Source: CAD feature listing. Evaluate the final solid. Frame: model axes, mm. Face numbers are marked on the shaded views. A direction names the side the tool comes from. Give positions to 0.01 mm unless a question says otherwise; leave off trailing zeros. Order: outer loops, then holes, each group sorted by start corner. A loop starts at its lowest first (then second) coordinate and runs counter-clockwise, first axis right, second up. Notation, with made-up numbers: M 55.25,18.5 L 85.25,18.5 A7 ccw 85.25,22.5 Z; hole C 1.5,57.5 d4. An arc over 180 degrees is marked long. Answer in a Markdown table with one row per item. Add a question column.
(1) Material intervals for line 1 along Y through (x, z) = (10, 4); line 2 along Y through (x, z) = (5.5, 7.25); line 3 along X through (y, z) = (-3.5, 5.75), sorted ascending.
(2) Mould query, pull axis Y, two halves, no side actions, for the marked faces 1, 2 and 3. Classes: pulls with the +Y half, pulls with the -Y half, needs draft (parallel to the pull), parting line crosses it, or undercut.
(3) Set-up query: the marked faces 4 and 5. Return all of +Z, -Z, +X, -X, +Y, -Y with unobstructed straight access to the full face (end or side cutting, diameter ignored); none if empty.
(4) Section query B-B, the plane x = -3.5. Return loops of the section in (y, z).
(5) Section query D-D, the plane x = -11.25. Return loops of the section in (y, z), plus the area to 3 significant figures.
(6) Section query C-C, the plane y = 12. Return loops of the section in (x, z).
(7) Pin query (flat end, axial travel): P1, Ø2.5, axis at x = 12, y = 12, coming from the -Z side. Return the tip coordinate at first contact, or that it passes through.
(8) Section query A-A, the plane z = 5. Return loops of the section in (x, y).
from build123d import *

# Parameters (mm, degrees)
F0_W     = 30
F0_H     = 30
F0_R     = 1.6
F1_DEPTH = 10.2


with BuildPart() as f1:
    # F0 (on Top) → F1 (new body)
    with BuildSketch(Plane.XY):
        Rectangle(F0_W, F0_H)
        with Locations((-12, -12)):
            Circle(F0_R, mode=Mode.SUBTRACT)
        with Locations((12, -12)):
            Circle(F0_R, mode=Mode.SUBTRACT)
        with Locations((-12, 12)):
            Circle(F0_R, mode=Mode.SUBTRACT)
        with BuildLine():
            ThreePointArc((13.0274698164, 6.366712667), (14.1270717478, 3.2673909823), (14.5, 0))
            ThreePointArc((14.5, 0), (10.6007075236, -9.8931794687), (1, -14.4654761415))
            Line((1, -14.4654761415), (1, -14.5))
            Line((1, -14.5), (0, -14.5))
            Line((0, -14.5), (-1, -14.5))
            Line((-1, -14.5), (-1, -14.4654761415))
            ThreePointArc((-1, -14.4654761415), (-12.5573683549, -7.25), (-13.0274698164, 6.366712667))
            Line((-13.0274698164, 6.366712667), (-13.0573683549, 6.3839745962))
            Line((-13.0573683549, 6.3839745962), (-12.5573697637, 7.2499975598))
            Line((-12.5573697637, 7.2499975598), (-12.0573683549, 8.1160254038))
            Line((-12.0573683549, 8.1160254038), (-12.0274698164, 8.0987634745))
            ThreePointArc((-12.0274698164, 8.0987634745), (0, 14.5), (12.0274698164, 8.0987634745))
            Line((12.0274698164, 8.0987634745), (12.0573683549, 8.1160254038))
            Line((12.0573683549, 8.1160254038), (12.5573697634, 7.2499975604))
            Line((12.5573697634, 7.2499975604), (13.0573683549, 6.3839745962))
            Line((13.0573683549, 6.3839745962), (13.0274698164, 6.366712667))
        make_face(mode=Mode.SUBTRACT)
        with Locations((12, 12)):
            Circle(F0_R, mode=Mode.SUBTRACT)
        with BuildLine():
            Line((6.9371965948, 2.850491783), (13.0274698164, 6.366712667))
            ThreePointArc((13.0274698164, 6.366712667), (12.8000410988, 6.8124113109), (12.5573697634, 7.2499975604))
            ThreePointArc((12.5573697634, 7.2499975604), (12.2997432975, 7.678952716), (12.0274698164, 8.0987634745))
            Line((12.0274698164, 8.0987634745), (5.9371965948, 4.5825425906))
            ThreePointArc((5.9371965948, 4.5825425906), (6.4951905284, 3.75), (6.9371965948, 2.850491783))
        make_face()
        with BuildLine():
            Line((-5.9371965948, 4.5825425906), (-12.0274698164, 8.0987634745))
            ThreePointArc((-12.0274698164, 8.0987634745), (-12.2997432977, 7.6789527158), (-12.5573697637, 7.2499975598))
            ThreePointArc((-12.5573697637, 7.2499975598), (-12.800041099, 6.8124113106), (-13.0274698164, 6.366712667))
            Line((-13.0274698164, 6.366712667), (-6.9371965948, 2.850491783))
            ThreePointArc((-6.9371965948, 2.850491783), (-6.4951905284, 3.75), (-5.9371965948, 4.5825425906))
        make_face()
        with BuildLine():
            ThreePointArc((0, -14.5), (0.5002978855, -14.4913664651), (1, -14.4654761415))
            Line((1, -14.4654761415), (1, -7.4330343737))
            ThreePointArc((1, -7.4330343737), (0, -7.5), (-1, -7.4330343737))
            Line((-1, -7.4330343737), (-1, -14.4654761415))
            ThreePointArc((-1, -14.4654761415), (-0.5002978855, -14.4913664651), (0, -14.5))
        make_face()
        with BuildLine():
            ThreePointArc((7.5, 0), (7.3579540112, 1.4527603965), (6.9371965948, 2.850491783))
            Line((6.9371965948, 2.850491783), (5.9371965948, 4.5825425906))
            ThreePointArc((5.9371965948, 4.5825425906), (0, 7.5), (-5.9371965948, 4.5825425906))
            Line((-5.9371965948, 4.5825425906), (-6.9371965948, 2.850491783))
            ThreePointArc((-6.9371965948, 2.850491783), (-6.4951905284, -3.75), (-1, -7.4330343737))
            Line((-1, -7.4330343737), (1, -7.4330343737))
            ThreePointArc((1, -7.4330343737), (5.6457948953, -4.9371044145), (7.5, 0))
        make_face()
        with BuildLine():
            ThreePointArc((12.5573697634, 7.2499975604), (12.8000410988, 6.8124113109), (13.0274698164, 6.366712667))
            Line((13.0274698164, 6.366712667), (13.0573683549, 6.3839745962))
            Line((13.0573683549, 6.3839745962), (12.5573697634, 7.2499975604))
        make_face()
        with BuildLine():
            ThreePointArc((-1, -7.4330343737), (0, -7.5), (1, -7.4330343737))
            Line((1, -7.4330343737), (-1, -7.4330343737))
        make_face()
        with BuildLine():
            Line((-6.9371965948, 2.850491783), (-5.9371965948, 4.5825425906))
            ThreePointArc((-5.9371965948, 4.5825425906), (-6.4951905284, 3.75), (-6.9371965948, 2.850491783))
        make_face()
        with BuildLine():
            Line((5.9371965948, 4.5825425906), (6.9371965948, 2.850491783))
            ThreePointArc((6.9371965948, 2.850491783), (6.4951905284, 3.75), (5.9371965948, 4.5825425906))
        make_face()
        with BuildLine():
            Line((1, -14.5), (1, -14.4654761415))
            ThreePointArc((1, -14.4654761415), (0.5002978855, -14.4913664651), (0, -14.5))
            Line((0, -14.5), (1, -14.5))
        make_face()
        with BuildLine():
            Line((-1, -14.5), (0, -14.5))
            ThreePointArc((0, -14.5), (-0.5002978855, -14.4913664651), (-1, -14.4654761415))
            Line((-1, -14.4654761415), (-1, -14.5))
        make_face()
        with BuildLine():
            Line((-13.0573683549, 6.3839745962), (-13.0274698164, 6.366712667))
            ThreePointArc((-13.0274698164, 6.366712667), (-12.800041099, 6.8124113106), (-12.5573697637, 7.2499975598))
            Line((-12.5573697637, 7.2499975598), (-13.0573683549, 6.3839745962))
        make_face()
        with BuildLine():
            ThreePointArc((-12.5573697637, 7.2499975598), (-12.2997432977, 7.6789527158), (-12.0274698164, 8.0987634745))
            Line((-12.0274698164, 8.0987634745), (-12.0573683549, 8.1160254038))
            Line((-12.0573683549, 8.1160254038), (-12.5573697637, 7.2499975598))
        make_face()
        with BuildLine():
            ThreePointArc((12.0274698164, 8.0987634745), (12.2997432975, 7.678952716), (12.5573697634, 7.2499975604))
            Line((12.5573697634, 7.2499975604), (12.0573683549, 8.1160254038))
            Line((12.0573683549, 8.1160254038), (12.0274698164, 8.0987634745))
        make_face()
    extrude(amount=F1_DEPTH)


solid = f1.part
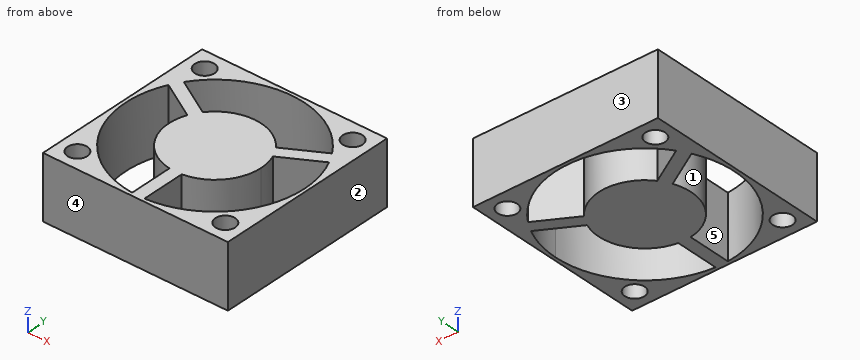
Values follow:
| question | item | result |
|---|---|---|
| 1 | line 1 | y = -15 to -10.5, 4.62 to 6.93, 10.5 to 15 |
| 1 | line 2 | y = -15 to -13.42, -5.1 to 5.1, 13.42 to 15 |
| 1 | line 3 | x = -15 to -14.07, -6.63 to 6.63, 14.07 to 15 |
| 2 | face 1 | undercut |
| 2 | face 2 | needs draft |
| 2 | face 3 | pulls with the +Y half |
| 3 | face 4 | +Z, -Z, +X, -X, -Y |
| 3 | face 5 | +Z, -Z |
| 4 | outline | M -15,0 L -14.07,0 L -14.07,10.2 L -15,10.2 Z; M -6.63,0 L 6.63,0 L 6.63,10.2 L -6.63,10.2 Z; M 14.07,0 L 15,0 L 15,10.2 L 14.07,10.2 Z |
| 5 | outline | M -15,0 L -13.41,0 L -13.41,10.2 L -15,10.2 Z; M -10.59,0 L -9.15,0 L -9.15,10.2 L -10.59,10.2 Z; M 5.34,0 L 7.65,0 L 7.65,10.2 L 5.34,10.2 Z; M 9.15,0 L 10.59,0 L 10.59,10.2 L 9.15,10.2 Z; M 13.41,0 L 15,0 L 15,10.2 L 13.41,10.2 Z |
| 5 | area | 85.3 mm² |
| 6 | outline | M -15,0 L -13.6,0 L -13.6,10.2 L -15,10.2 Z; M -10.4,0 L -8.14,0 L -8.14,10.2 L -10.4,10.2 Z; M 8.14,0 L 10.4,0 L 10.4,10.2 L 8.14,10.2 Z; M 13.6,0 L 15,0 L 15,10.2 L 13.6,10.2 Z |
| 7 | P1 | passes through |
| 8 | outline | M -15,-15 L 15,-15 L 15,15 L -15,15 Z; hole C -12,-12 d3.2; hole C -12,12 d3.2; hole M -13.03,6.37 A14.5 ccw -1,-14.47 L -1,-7.43 A7.5 cw -6.94,2.85 Z; hole M -12.03,8.1 L -5.94,4.58 A7.5 cw 5.94,4.58 L 12.03,8.1 A14.5 ccw Z; hole M 1,-14.47 A14.5 ccw 13.03,6.37 L 6.94,2.85 A7.5 cw 1,-7.43 Z; hole C 12,-12 d3.2; hole C 12,12 d3.2 |
